Verification items for the finished model (mm, model axes). Face numbers are marked on the shaded views. A direction names the side the tool comes from. Round coordinates to 2 decimals unless told otherwise and drop trailing zeros. Write each loop counter-clockwise with the first axis right and the second up, starting at its lowest first coordinate (ties: lowest second). Pieces come first, ordered by that corner, then holes. Notation, with made-up numbers: (-18.5, 59) -> (33.5, 59) arc R17 ccw to (33.5, 67) -> close; hole circle Ø5 at (-31, 35). An arc over 180 degrees is marked (long way). Answer as a JSON object with one key per item and string values. Group by question number.
(1) Gauge pin test, flat ends, axial feed: pin 1 Ø1.5 at (y, z) = (-1, 25.5) entering from +X; pin 2 Ø1.5 at (x, y) = (-8.5, -1.5) entering from +Z; pin 3 Ø14 at (x, z) = (-10, 5.5) entering from -Y; pin 4 Ø2.5 at (y, z) = (-15.9, 41.11) entering from -X. Record the tip position at first contact, or that the pin passes through.
(2) Set-up check for the marked faces 1 and 2: record each of +Z, -Z, +X, -X, +Y, -Y from which the full face is reachable in a straight line by a thin tool's end or side.
(3) Draft check along X on the marked faces 3, 4 and 5. Enter one of: released by +X, released by -X, zero draft, split by the parting line, or undercut.
(4) Sectioned sample at C-C on y = -2. Record the cut outline in (x, z).
(5) Sectioned sample at B-B on y = -13. Record the cut outline in (x, z).
(6) Sectioned sample at D-D on z = 3. Record the cut outline in (x, y).
(7) Sectioned sample at A-A on z = 29. Record the cut outline in (x, y).
(8) Scan lines: L1, parallel to X at y = -6.5, z = 37; L2, parallel to Y at x = -0.5, z = -1; L3, parallel to X at y = -4.25, z = -3.5. Record each from-to range of solid material in increasing order. Write a range as from..to.
```python
from build123d import *

# Parameters (mm, degrees)
SKETCH1_W                      = 32
SKETCH1_H                      = 60
BASE_FLANGE1_DEPTH             = 3
EDGE_FLANGE1_STRIP_W           = 16
EDGE_FLANGE1_STRIP_H           = 3
EDGE_FLANGE1_STRIP_CUT_DEPTH   = 60
EDGE_FLANGE1_STRIP_2_W         = 16
EDGE_FLANGE1_STRIP_2_H         = 3
EDGE_FLANGE1_STRIP_CUT_2_DEPTH = 60
EDGE_FLANGE1_DEPTH             = 60
EDGE_FLANGE1_BEND_DEPTH        = 60
SKETCH18_R                     = 1
SKETCH18_W                     = 24
SKETCH18_H                     = 13
CUT_EXTRUDE1_DEPTH             = 68.01070511
SKETCH19_W                     = 20
SKETCH19_H                     = 40
CUT_EXTRUDE2_DEPTH             = 60.604400839
SKETCH20_W                     = 24
SKETCH20_H                     = 2.600711811
CUT_EXTRUDE3_DEPTH             = 68.01070511


# Sheet-metal steps are written as plain solids
with BuildPart() as part:
    # Sketch1 → Base-Flange1 (new body)
    with BuildSketch(Plane(origin=(0, 0, 0), x_dir=(1, 0, 0), z_dir=(0, 1, 0))):
        with Locations((-3.5, -19.208074534)):
            Rectangle(SKETCH1_W, SKETCH1_H)
    extrude(amount=-BASE_FLANGE1_DEPTH)

    # Edge-Flange1 strip (across the edge) → Edge-Flange1 strip cut (cut)
    with BuildSketch(Plane(origin=(12.5, -3, -10.791925466), x_dir=(-1, 0, 0), z_dir=(0, 0, 1))):
        with Locations((-6, -1.5)):
            Rectangle(EDGE_FLANGE1_STRIP_W, EDGE_FLANGE1_STRIP_H)
    extrude(amount=EDGE_FLANGE1_STRIP_CUT_DEPTH, mode=Mode.SUBTRACT)

    # Edge-Flange1 strip 2 (across the edge) → Edge-Flange1 strip cut 2 (cut)
    with BuildSketch(Plane(origin=(-19.5, -3, 49.208074534), x_dir=(1, 0, 0), z_dir=(0, 0, -1))):
        with Locations((-6, -1.5)):
            Rectangle(EDGE_FLANGE1_STRIP_2_W, EDGE_FLANGE1_STRIP_2_H)
    extrude(amount=EDGE_FLANGE1_STRIP_CUT_2_DEPTH, mode=Mode.SUBTRACT)

    # Edge-Flange1 section (across the edge) → Edge-Flange1 (add)
    with BuildSketch(Plane(origin=(12.5, -3, -10.791925466), x_dir=(-1, 0, 0), z_dir=(0, 0, 1))):
        with BuildLine():
            Line((-3, 2), (-3, 22))
            Line((-3, 22), (0, 22))
            Line((0, 22), (0, 2))
            ThreePointArc((0, 2), (0.585786438, 0.585786438), (2, 0))
            Line((2, 0), (2, -3))
            ThreePointArc((2, -3), (-1.535533906, -1.535533906), (-3, 2))
        make_face()
    extrude(amount=EDGE_FLANGE1_DEPTH)

    # Edge-Flange1 section 2 (across the edge) → Edge-Flange1 bend (add)
    with BuildSketch(Plane(origin=(-19.5, -3, 49.208074534), x_dir=(1, 0, 0), z_dir=(0, 0, -1))):
        with BuildLine():
            Line((-3, 2), (-3, 22))
            Line((-3, 22), (0, 22))
            Line((0, 22), (0, 2))
            ThreePointArc((0, 2), (0.585786438, 0.585786438), (2, 0))
            Line((2, 0), (2, -3))
            ThreePointArc((2, -3), (-1.535533906, -1.535533906), (-3, 2))
        make_face()
    extrude(amount=EDGE_FLANGE1_BEND_DEPTH)

    # Sketch18 → Cut-Extrude1 (cut, through all)
    with BuildSketch(Plane(origin=(15.5, 0, 0), x_dir=(0, 0, -1), z_dir=(1, 0, 0))):
        with Locations(Location((-41.108074534, -15.899288189, 0), (0, 0, 90))):
            Circle(SKETCH18_R)
        with Locations(Location((-13.308074534, -15.899288189, 0), (0, 0, 90))):
            Circle(SKETCH18_R)
        with Locations((-27.208074534, -15.899288189)):
            Rectangle(SKETCH18_W, SKETCH18_H)
    extrude(amount=-CUT_EXTRUDE1_DEPTH, mode=Mode.SUBTRACT)

    # Sketch19 → Cut-Extrude2 (cut, through all)
    with BuildSketch(Plane(origin=(0, 0, 0), x_dir=(1, 0, 0), z_dir=(0, 1, 0))):
        with Locations((-3.5, -29.208074534)):
            Rectangle(SKETCH19_W, SKETCH19_H)
    extrude(amount=-CUT_EXTRUDE2_DEPTH, mode=Mode.SUBTRACT)

    # Sketch20 → Cut-Extrude3 (cut, through all)
    with BuildSketch(Plane(origin=(15.5, 0, 0), x_dir=(0, 0, -1), z_dir=(1, 0, 0))):
        with Locations((-27.208074534, -23.699644095)):
            Rectangle(SKETCH20_W, SKETCH20_H)
    extrude(amount=-CUT_EXTRUDE3_DEPTH, mode=Mode.SUBTRACT)


solid = part.part
```
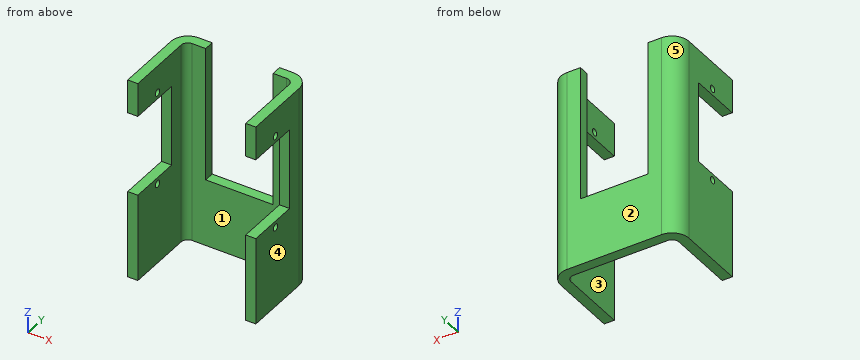
Computed values:
{
 "1": {"pin 1": "x = 14.3", "pin 2": "z = 9.21", "pin 3": "y = -3", "pin 4": "x = -22.5"},
 "2": {"face 1": "+Z, -Z, -Y", "face 2": "+Z, -Z, +X, -X, +Y"},
 "3": {"face 3": "undercut", "face 4": "released by +X", "face 5": "released by -X"},
 "4": {"outline": "(-21.5, -10.79) -> (14.5, -10.79) -> (14.5, 49.21) -> (6.5, 49.21) -> (6.5, 9.21) -> (-13.5, 9.21) -> (-13.5, 49.21) -> (-21.5, 49.21) -> close"},
 "5": {"outline": "(-22.5, -10.79) -> (-19.5, -10.79) -> (-19.5, 15.21) -> (-22.5, 15.21) -> close; (-22.5, 39.21) -> (-19.5, 39.21) -> (-19.5, 49.21) -> (-22.5, 49.21) -> close; (12.5, -10.79) -> (15.5, -10.79) -> (15.5, 15.21) -> (12.5, 15.21) -> close; (12.5, 39.21) -> (15.5, 39.21) -> (15.5, 49.21) -> (12.5, 49.21) -> close"},
 "6": {"outline": "(-22.5, -25) -> (-19.5, -25) -> (-19.5, -5) arc R2 cw to (-17.5, -3) -> (10.5, -3) arc R2 cw to (12.5, -5) -> (12.5, -25) -> (15.5, -25) -> (15.5, -5) arc R5 ccw to (10.5, 0) -> (-17.5, 0) arc R5 ccw to (-22.5, -5) -> close"},
 "7": {"outline": "(-22.5, -9.4) -> (-19.5, -9.4) -> (-19.5, -5) arc R2 cw to (-17.5, -3) -> (-13.5, -3) -> (-13.5, 0) -> (-17.5, 0) arc R5 ccw to (-22.5, -5) -> close; (6.5, -3) -> (10.5, -3) arc R2 cw to (12.5, -5) -> (12.5, -9.4) -> (15.5, -9.4) -> (15.5, -5) arc R5 ccw to (10.5, 0) -> (6.5, 0) -> close"},
 "8": {"L1": "-22.5..-19.5, 12.5..15.5", "L2": "-3..0", "L3": "-22.44..-19.35, 12.35..15.44"}
}
